Job drawing, mm, ordinate dimensions from the low corner. One solid piece. Give positions to 0.01 mm unless a question says otherwise; leave off trailing zeros. Loops run counter-clockwise (first coordinate to the right, second up) from the corner with the lowest first, then second, coordinate; pieces in that order, holes last. Notation, with made-up numbers: (52.25, 55) - (66.25, 55) arc R15 cw to (66.25, 71) - close; hole circle Ø6 at (32, 17). An arc over 180 degrees is marked (long way). Use a Markdown table: item, result.
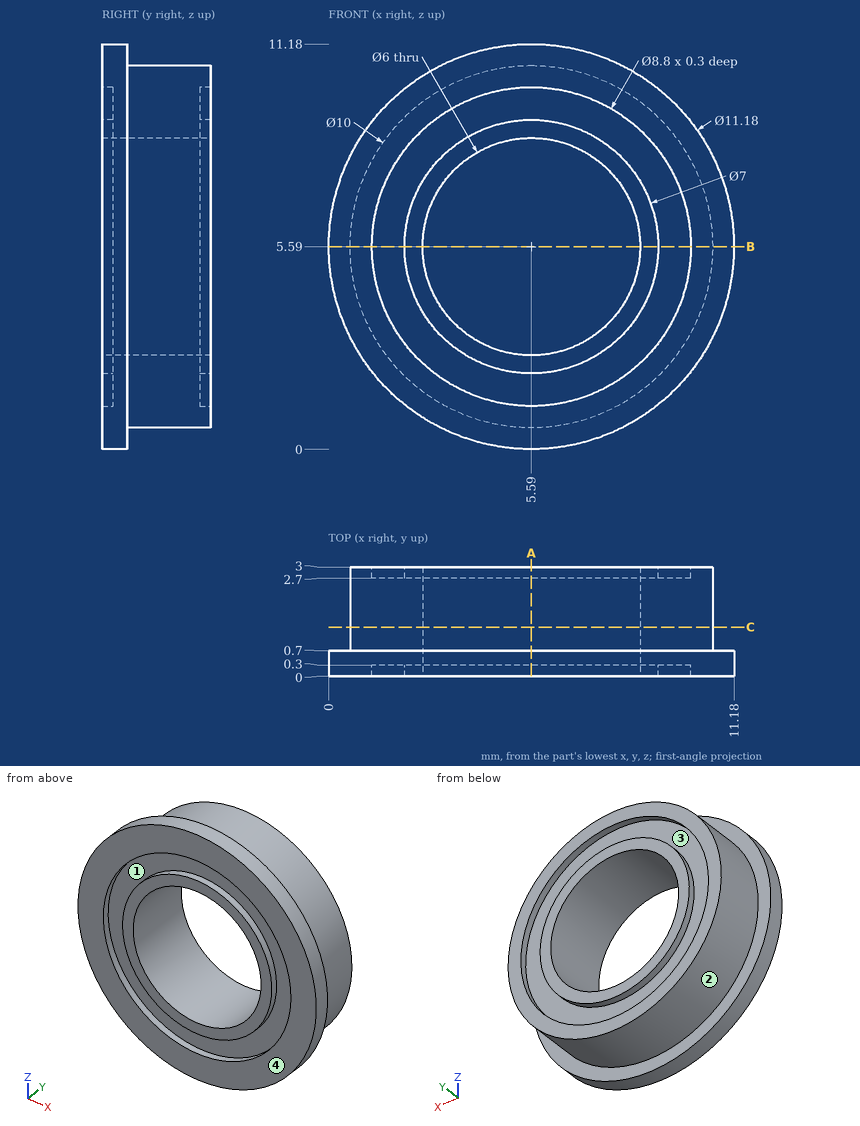
(1) Drill centre lines: probe 1 along X at (y, z) = (0.25, 5.59); probe 2 along Z at (x, y) = (5.5, 1.4). Where is each one in solid material? Low to high. Write a range as [from, to].
Computed:
| item | result |
|---|---|
| probe 1 | [0, 1.19], [2.09, 2.59], [8.59, 9.09], [9.99, 11.18] |
| probe 2 | [0.59, 2.59], [8.59, 10.59] |
(2) Slice it at A-A, the plane x = 5.59. Write the cut outline in (y, z).
Computed:
| item | result |
|---|---|
| outline | (0, 0) - (0.7, 0) - (0.7, 0.59) - (3, 0.59) - (3, 1.19) - (2.7, 1.19) - (2.7, 2.09) - (3, 2.09) - (3, 2.59) - (0, 2.59) - (0, 2.09) - (0.3, 2.09) - (0.3, 1.19) - (0, 1.19) - close; (0, 8.59) - (3, 8.59) - (3, 9.09) - (2.7, 9.09) - (2.7, 9.99) - (3, 9.99) - (3, 10.59) - (0.7, 10.59) - (0.7, 11.18) - (0, 11.18) - (0, 9.99) - (0.3, 9.99) - (0.3, 9.09) - (0, 9.09) - close |
(3) Mould opens along Z. For the marked faces 1, 2, 3 and 4 say: pulls with the +Z half, pulls with the -Z half, needs draft (parallel to the pull), parting line crosses it, or undercut.
Computed:
| item | result |
|---|---|
| face 1 | undercut |
| face 2 | parting line crosses it |
| face 3 | undercut |
| face 4 | needs draft |
(4) Slice it at B-B, the plane z = 5.59. Write the cut outline in (x, y).
Computed:
| item | result |
|---|---|
| outline | (0, 0) - (1.19, 0) - (1.19, 0.3) - (2.09, 0.3) - (2.09, 0) - (2.59, 0) - (2.59, 3) - (2.09, 3) - (2.09, 2.7) - (1.19, 2.7) - (1.19, 3) - (0.59, 3) - (0.59, 0.7) - (0, 0.7) - close; (8.59, 0) - (9.09, 0) - (9.09, 0.3) - (9.99, 0.3) - (9.99, 0) - (11.18, 0) - (11.18, 0.7) - (10.59, 0.7) - (10.59, 3) - (9.99, 3) - (9.99, 2.7) - (9.09, 2.7) - (9.09, 3) - (8.59, 3) - close |
(5) Slice it at C-C, the plane y = 1.35. Write the cut outline in (x, z), plus the area to 3 significant figures.
Computed:
| item | result |
|---|---|
| outline | circle Ø10 at (5.59, 5.59); hole circle Ø6 at (5.59, 5.59) |
| area | 50.3 mm² |
(6) Pin check, flat tip, straight feed: P1, Ø4, axis at x = 5, z = 9, coming from the -Y side. Stop position of the tip, or through.
Computed:
| item | result |
|---|---|
| P1 | y = 0 |
